```python
from build123d import *

# Parameters (mm, degrees)
SKETCH1_W           = 65.37
SKETCH1_H           = 19.19
BOSS_EXTRUDE1_DEPTH = 22.27
SKETCH2_R           = 2.665
BOSS_EXTRUDE2_DEPTH = 9.32


with BuildPart() as part:
    # Sketch1 → Boss-Extrude1 (new body)
    with BuildSketch(Plane.XY):
        with Locations((32.685, 9.595)):
            Rectangle(SKETCH1_W, SKETCH1_H)
    extrude(amount=-BOSS_EXTRUDE1_DEPTH)

    # Sketch2 → Boss-Extrude2 (add)
    with BuildSketch(Plane.XZ):
        with Locations((55.37, -11.135)):
            Circle(SKETCH2_R)
    extrude(amount=BOSS_EXTRUDE2_DEPTH)


solid = part.part
```
Input: part model. Units: mm. Frame: model coordinates. A direction names the side the tool comes from. Give positions to 0.01 mm unless a question says otherwise; leave off trailing zeros. Order: outer loops, then holes, each group sorted by start corner. A loop starts at its lowest first (then second) coordinate and runs counter-clockwise, first axis right, second up. Notation, with made-up numbers: M 2,22 L 39,22 A12 cw 39,30 Z; hole C 39.5,-24.75 d11. An arc over 180 degrees is marked long. Return JSON: item names as keys, results as strings.
Item 1: Cut plane A-A (x = 55.37). Return loops of the section in (y, z), then the cut area to 3 significant figures.
Solutions:
{"outline": "M -9.32,-13.8 L 0,-13.8 L 0,-22.27 L 19.19,-22.27 L 19.19,0 L 0,0 L 0,-8.47 L -9.32,-8.47 Z", "area": "477 mm^2"}
Item 2: First-contact query: P1, Ø6, axis at x = 23.5, z = -12.5, coming from the -Y side. Flat tip, straight axial feed; report the tip coordinate or a pass-through.
Solutions:
{"P1": "y = 0"}
Item 3: Access query for faces 1 (the cylindrical face through (57.9, -4.6, -10.3)), 2 (the flat face through (32, 19.19, -11)). Directions: +Z, -Z, +X, -X, +Y, -Y. A direction counts if a zero-diameter tool reaches every point of the face in a straight line with its end or side. Return the directions, or none.
Solutions:
{"face 1": "-Y", "face 2": "+Z, -Z, +X, -X, +Y"}
Item 4: Cut plane C-C (z = -16.5). Return loops of the section in (x, y), then the cut area to 3 significant figures.
Solutions:
{"outline": "M 0,0 L 65.37,0 L 65.37,19.19 L 0,19.19 Z", "area": "1,250 mm^2"}
Item 5: Ray query, probe 1 along Y at (x, z) = (17.5, -15.5); probe 2 along X at (y, z) = (-2, -9.5); probe 3 along Z at (x, y) = (57.5, -0.75). Return the intervals inside material, ascending.
Solutions:
{"probe 1": "0 to 19.19", "probe 2": "53.27 to 57.47", "probe 3": "-12.74 to -9.53"}
Item 6: Cut plane D-D (x = 18). Return loops of the section in (y, z).
Solutions:
{"outline": "M 0,-22.27 L 19.19,-22.27 L 19.19,0 L 0,0 Z"}
Item 7: Cut plane B-B (z = -10.5). Return loops of the section in (x, y).
Solutions:
{"outline": "M 0,0 L 52.78,0 L 52.78,-9.32 L 57.96,-9.32 L 57.96,0 L 65.37,0 L 65.37,19.19 L 0,19.19 Z"}
